Work out the finished part from the listing and answer in its coordinate system (mm). Give positions to 0.01 mm unless a question says otherwise; leave off trailing zeros. Loops run counter-clockwise (first coordinate to the right, second up) from the corner with the lowest first, then second, coordinate; pieces in that order, holes last. Notation, with made-up numbers: (18.5, -21.5) - (54.5, -21.5) arc R27 ccw to (54.5, 7.5) - close; hole circle Ø2 at (27, 27.5). An arc over 180 degrees is marked (long way). Use CSV: the item, a comma, the result in double quotes.
Autodesk Inventor part; units mm, degrees
ref_plane "YZ Plane" through (0, 0, 0) normal (1, 0, 0) x (0, 1, 0)
ref_plane "XZ Plane" through (0, 0, 0) normal (0, 1, 0) x (-1, 0, 0)
ref_plane "XY Plane" through (0, 0, 0) normal (0, 0, 1) x (1, 0, 0)
sketch "Sketch1" plane through (0, 0, 0) normal (0, 0, 1) x (1, 0, 0)
  line L0 (-28, 0) -> (28, 0)
  line L1 (0, -12) -> (0, 72)
  line L2 (-20, 60) -> (20, 60)
  line L3 (20, 60) -> (20, 0)
  line L4 (20, 0) -> (-20, 0)
  line L5 (-20, 0) -> (-20, 60)
  arc A0 (20, 40) -> (-20, 40) centre (0, 40) ccw
  line L6 (-20, 40) -> (20, 40) construction
  circle A1 centre (0, 40) radius 8
  point P0 (0, 0)
  point P1 (0, 60)
  point P2 (0, 0)
  dimension "d0" = 40
  dimension "d1" = 60
  dimension "d2" = 8
extrude "Extrusion1" add sketch "Sketch1" along normal mid plane 24 contours L5 A0 L1 A1 L0 | L1 A1 A0 L3 L0
fillet "Fillet1" radius 2 8 edges at (20, 20, 12) (-14.1421, 54.1421, 12) (14.1421, 54.1421, 12) (-20, 20, 12) (20, 20, -12) (-14.1421, 54.1421, -12) (14.1421, 54.1421, -12) (-20, 20, -12)
properties part number "Lagar"
Item 1: A cutting plane is placed at B-B on z = 4.5. Determine the outline of the cut face in (x, y), and give its area (3 significant figures).
Determined:
outline,"(-20, 0) - (20, 0) - (20, 40) arc R20 ccw to (-20, 40) - close; hole circle Ø16 at (0, 40)"
area,"2,030 mm²"
Item 2: Given P1, Ø12, axis at y = 53, z = -6, coming from the +X side (3 decimals); P2, Ø2, axis at x = 9.5, z = 6, coming from the +Y side; P3, Ø18.5, axis at x = 0, y = 40, coming from the -Z side; P4, Ø6, axis at y = 48, z = -6, coming from the +X side, each flat-ended and moving along its own axis, determine where each tip first touches the part or whether it passes through.
Determined:
P1,"stops at x = 18.735"
P2,"stops at y = 58.1"
P3,"stops at z = -12"
P4,"stops at x = 19.36"
Item 3: The mould has two halves that part along X. Classify faces 1 (the cylindrical face through (-1.041, 47.932, 0.168)), 2 (the cylindrical face through (-19.43, 20.28, 11.4)), 3 (the flat face through (0, 29, 12)): pulls with the +X half, pulls with the -X half, needs draft (parallel to the pull), parting line crosses it, or undercut.
Determined:
face 1,"undercut"
face 2,"pulls with the -X half"
face 3,"needs draft"
Item 4: A cutting plane is placed at C-C on y = 36. Determine the outline of the cut face in (x, z), and give its area (3 significant figures).
Determined:
outline,"(-20, -10) arc R2 ccw to (-18, -12) - (-6.93, -12) - (-6.93, 12) - (-18, 12) arc R2 ccw to (-20, 10) - close; (6.93, -12) - (18, -12) arc R2 ccw to (20, -10) - (20, 10) arc R2 ccw to (18, 12) - (6.93, 12) - close"
area,"624 mm²"
Item 5: A cutting plane is placed at A-A on x = 0. Determine the outline of the cut face in (y, z), and give its area (3 significant figures).
Determined:
outline,"(0, -12) - (32, -12) - (32, 12) - (0, 12) - close; (48, -12) - (58, -12) arc R2 ccw to (60, -10) - (60, 10) arc R2 ccw to (58, 12) - (48, 12) - close"
area,"1,050 mm²"
Item 6: Find the intervals of material crossed by line 1 (Y direction, x = 0, z = -2); line 2 (X direction, y = 40.5, z = -1.25); line 3 (Y direction, x = -1.5, z = 11.25), in increasing order.
Determined:
line 1,"y = 0 to 32, 48 to 60"
line 2,"x = -19.99 to -7.98, 7.98 to 19.99"
line 3,"y = 0 to 32.14, 47.86 to 59.5"
